Check sheet for the modelled part. Datum: model origin and axes. Units: mm. Round coordinates to 2 decimals unless told otherwise and drop trailing zeros. Loops run counter-clockwise (first coordinate to the right, second up) from the corner with the lowest first, then second, coordinate; pieces in that order, holes last. Notation, with made-up numbers: (-37.5, 56.5) - (-29.5, 56.5) arc R18 ccw to (-29.5, 65.5) - close; hole circle Ø2 at (7, 70.25). An arc over 180 degrees is marked (long way). Return JSON: item names as keys, results as strings.
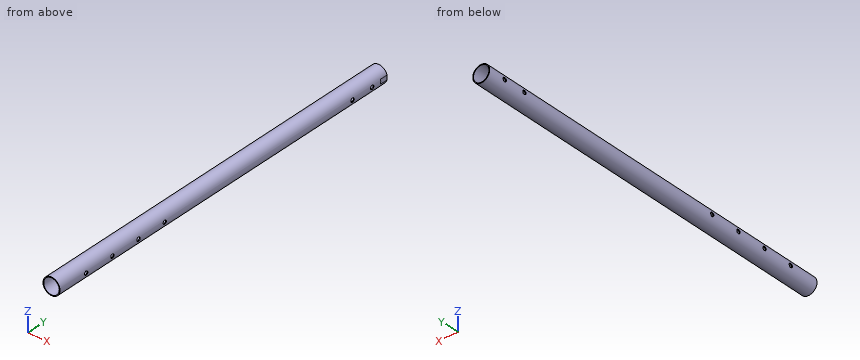
from build123d import *

# Parameters (mm, degrees)
SKETCH1_R               = 11
SKETCH1_R_2             = 10
BOSS_EXTRUDE1_DEPTH     = 500
SKETCH2_W               = 0.79991629
SKETCH2_H               = 5.878473502
CUT_EXTRUDE1_DEPTH      = 10
CUT_EXTRUDE2_DEPTH      = 501.587216984
CUT_EXTRUDE2_DEPTH_BACK = 501.587216984
SKETCH3_R               = 2.5
CUT_EXTRUDE3_DEPTH      = 501.587217091
CUT_EXTRUDE3_DEPTH_BACK = 501.587217091
SKETCH5_R               = 2.5


with BuildPart() as part:
    # Sketch1 → Boss-Extrude1 (new body)
    with BuildSketch(Plane(origin=(0, 0, 0), x_dir=(1, 0, 0), z_dir=(0, 1, 0))):
        with Locations(Location((0, 0, 0), (0, 0, 270))):
            Circle(SKETCH1_R)
        with Locations(Location((0, 0, 0), (0, 0, 270))):
            Circle(SKETCH1_R_2, mode=Mode.SUBTRACT)
    extrude(amount=BOSS_EXTRUDE1_DEPTH)

    # Sketch2 → Cut-Extrude1 (cut)
    with BuildSketch(Plane(origin=(0, 500, 0), x_dir=(1, 0, 0), z_dir=(0, 1, 0))):
        with Locations((11, 0)):
            Rectangle(SKETCH2_W, SKETCH2_H)
    extrude(amount=-CUT_EXTRUDE1_DEPTH, mode=Mode.SUBTRACT)

    # Sketch3 → Cut-Extrude2 (cut, two sides: drawn at the far end of the back side and taken through both)
    with BuildSketch(Plane(origin=(10.600041855, 0, 0), x_dir=(0, 0, -1), z_dir=(1, 0, 0)).offset(-CUT_EXTRUDE2_DEPTH_BACK)):
        with Locations((0, 477)):
            Circle(SKETCH3_R)
        with Locations((0, 447)):
            Circle(SKETCH3_R)
    extrude(amount=CUT_EXTRUDE2_DEPTH + CUT_EXTRUDE2_DEPTH_BACK, mode=Mode.SUBTRACT)

    # Sketch5 → Cut-Extrude3 (cut, two sides: drawn at the far end of the back side and taken through both)
    with BuildSketch(Plane(origin=(10.600041855, 0, 0), x_dir=(0, 0, -1), z_dir=(1, 0, 0)).offset(-CUT_EXTRUDE3_DEPTH_BACK)):
        with Locations((0, 40)):
            Circle(SKETCH5_R)
        with Locations((0, 80)):
            Circle(SKETCH5_R)
        with Locations((0, 120)):
            Circle(SKETCH5_R)
        with Locations((0, 160)):
            Circle(SKETCH5_R)
    extrude(amount=CUT_EXTRUDE3_DEPTH + CUT_EXTRUDE3_DEPTH_BACK, mode=Mode.SUBTRACT)


solid = part.part
Q1. Depth check by flat-ended pin: P1, Ø1, axis at y = 300.5, z = -5.5, coming from the +X side; P2, Ø1.8, axis at y = 493, z = -1, coming from the +X side; P3, Ø12, axis at x = 6.5, y = 291, coming from the +Z side. Enter the tip coordinate at first touch or a pass-through.
Answer key:
{"P1": "stops at x = 9.8", "P2": "stops at x = 10.6", "P3": "stops at z = 10.99"}
Q2. Scan lines: probe 1 along X at (y, z) = (346, -0.5); probe 2 along X at (y, z) = (209, 4.25); probe 3 along Z at (x, y) = (2.75, 80.5). Record each from-to range of solid material in increasing order. Write a range as [from, to].
Answer key:
{"probe 1": "x = [-10.99, -9.99], [9.99, 10.99]", "probe 2": "x = [-10.15, -9.05], [9.05, 10.15]", "probe 3": "z = [-10.65, -9.61], [9.61, 10.65]"}
Q3. Sectioned sample at C-C (y = 183.5). Enter the section's corners in (x, z).
Answer key:
{"outline": "circle Ø22 at (0, 0); hole circle Ø20 at (0, 0)"}
Q4. Sectioned sample at A-A (x = 0). Enter the section's corners in (y, z), plus the area to 3 significant figures.
Answer key:
{"outline": "(0, -11) - (500, -11) - (500, -10) - (0, -10) - close; (0, 10) - (500, 10) - (500, 11) - (0, 11) - close", "area": "1,000 mm²"}
Q5. Sectioned sample at B-B (z = -6.5). Enter the section's corners in (x, y).
Answer key:
{"outline": "(-8.87, 0) - (-7.6, 0) - (-7.6, 500) - (-8.87, 500) - close; (7.6, 0) - (8.87, 0) - (8.87, 500) - (7.6, 500) - close"}
